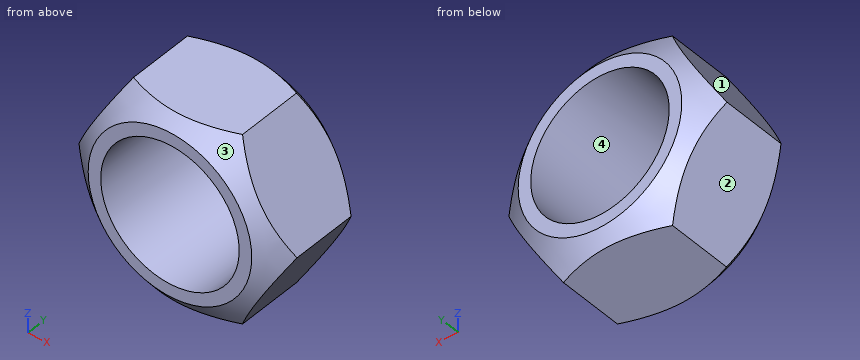
```python
from build123d import *

# Parameters (mm, degrees)
SKETCH1_R           = 6.35
BOSS_EXTRUDE1_DEPTH = 10


with BuildPart() as part:
    # Sketch1 → Boss-Extrude1 (new body)
    with BuildSketch(Plane(origin=(0, 0, 0), x_dir=(1, 0, 0), z_dir=(0, 1, 0))):
        Polygon((10, 0), (5, 8.660254038), (-5, 8.660254038), (-10, 0), (-5, -8.660254038), (5, -8.660254038), align=None)
        with Locations(Location((0, 0, 0), (0, 0, 270))):
            Circle(SKETCH1_R, mode=Mode.SUBTRACT)
    extrude(amount=BOSS_EXTRUDE1_DEPTH)

    # Sketch3 → Cut-Revolve1 (revolve, cut)
    with BuildSketch(Plane.XY, mode=Mode.PRIVATE) as cut_revolve1_sk:
        Polygon((-10, 10), (-10, 7.996913118), (-7.5, 10), align=None)
    cut_revolve1 = revolve(cut_revolve1_sk.sketch.rotate(Axis((0, 10, 0), (0, -1, 0)), 60.000000094), axis=Axis((0, 10, 0), (0, -1, 0)), mode=Mode.SUBTRACT)

    # Mirror1: Cut-Revolve1 across plane
    add(cut_revolve1.mirror(Plane(origin=(0, 5, 0), x_dir=(0, 0, 1), z_dir=(0, -1, 0))), mode=Mode.SUBTRACT)


solid = part.part
```
Design review of the part built by this model. Coordinates are the model's own, in mm. Face numbers are marked on the shaded views. Round coordinates to 2 decimals unless told otherwise and drop trailing zeros. Order: outer loops, then holes, each group sorted by start corner. A loop starts at its lowest first (then second) coordinate and runs counter-clockwise, first axis right, second up. Notation, with made-up numbers: M -28,-15 L -18,-15 A11 cw -18,3 Z; hole C -32,34.5 d1. An arc over 180 degrees is marked long. Put each result on its own line as item: value.
Q1. Consider section A-A (x = 0). State the section outline as (y, z) points, and give its area (3 significant figures).
Reported:
outline: M 0,-7.5 L 0.93,-8.66 L 9.07,-8.66 L 10,-7.5 L 10,-6.35 L 0,-6.35 Z; M 0,6.35 L 10,6.35 L 10,7.5 L 9.07,8.66 L 0.93,8.66 L 0,7.5 Z
area: 44.0 mm²
Q2. Draft analysis for pull direction Z (two halves, no side actions). For the marked faces 1, 2, 3 and 4, state which applies: released by +Z, released by -Z, zero draft, split by the parting line, or undercut.
Reported:
face 1: released by +Z
face 2: released by -Z
face 3: split by the parting line
face 4: undercut
Q3. Insertion check: pin 1 Ø1 at (x, z) = (-4.5, -0.5) entering from +Y; pin 2 Ø5 at (y, z) = (4, -2) entering from +X; pin 3 Ø1.5 at (x, y) = (6, 4) entering from -Z. Each pin has a flat end and moves straight along its axis. Give the tip position at first contact, or say it passes through.
Reported:
pin 1: through
pin 2: x = 10
pin 3: z = -8.23
Q4. To check wall thickness, follow line 1 (X direction, y = 4.5, z = 2); line 2 (X direction, y = 1.5, z = 2.75); line 3 (Z direction, x = -5, y = 9). State the ranges of each line that lie inside material, in increasing order.
Reported:
line 1: -8.85 to -6.03, 6.03 to 8.85
line 2: -8.41 to -5.72, 5.72 to 8.41
line 3: -7.18 to -3.91, 3.91 to 7.18
Q5. Consider section B-B (y = 7.75). State the section outline as (x, z) points, and give its area (3 significant figures).
Reported:
outline: M -10,0 L -5,-8.66 L 5,-8.66 L 10,0 L 5,8.66 L -5,8.66 Z; hole C 0,0 d12.7
area: 133 mm²
